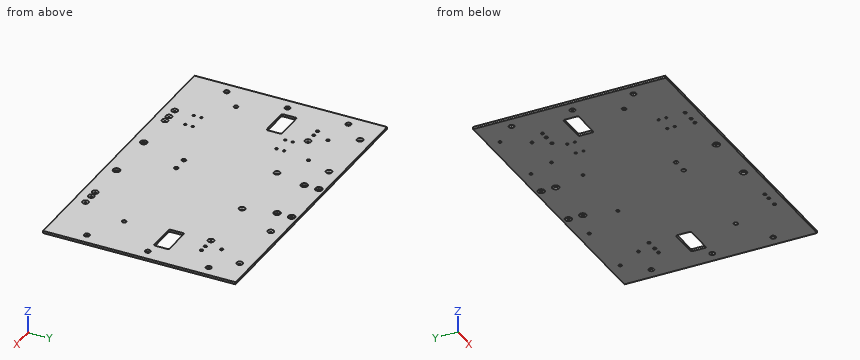
```python
from build123d import *

# Parameters (mm, degrees)
SKETCH_1_W          = 390
SKETCH_1_H          = 253
EXTRUDE_1_DEPTH     = 3
SKETCH_3_R          = 4.5
SKETCH_3_R_2        = 3.5
SKETCH_3_R_3        = 2.75
SKETCH_3_R_4        = 2
SKETCH_3_R_5        = 1.5
CUT_EXTRUDE_3_DEPTH = 233.456985268
SKETCH_5_W          = 40
SKETCH_5_H          = 20
CUT_EXTRUDE_4_DEPTH = 233.456985268
FILLET_1_R          = 2
CHAMFER_1_SIZE      = 2


with BuildPart() as part:
    # 草图1 → 凸台-拉伸1 (new body)
    with BuildSketch(Plane.XY):
        Rectangle(SKETCH_1_W, SKETCH_1_H)
    extrude(amount=EXTRUDE_1_DEPTH)

    # 草图3 → 切除-拉伸3 (cut, through all)
    with BuildSketch(Plane.XY):
        with Locations((-35, -111.5)):
            Circle(SKETCH_3_R)
        with Locations((35, -111.5)):
            Circle(SKETCH_3_R)
        with Locations((-180, -76.5)):
            Circle(SKETCH_3_R_2)
        with Locations(Location((180, -76.5, 0), (0, 0, 180))):
            Circle(SKETCH_3_R_2)
        with Locations((-35, 118.5)):
            Circle(SKETCH_3_R)
        with Locations(Location((35, 118.5, 0), (0, 0, 180))):
            Circle(SKETCH_3_R)
        with Locations((-35, 99.5)):
            Circle(SKETCH_3_R)
        with Locations(Location((35, 99.5, 0), (0, 0, 180))):
            Circle(SKETCH_3_R)
        with Locations((-155, -51.5)):
            Circle(SKETCH_3_R_3)
        with Locations((-21, -51.5)):
            Circle(SKETCH_3_R_3)
        with Locations((-1, -51.5)):
            Circle(SKETCH_3_R_3)
        with Locations((133, -51.5)):
            Circle(SKETCH_3_R_3)
        with Locations((-149.5, 58.5)):
            Circle(SKETCH_3_R_4)
        with Locations((-139.5, 58.5)):
            Circle(SKETCH_3_R_4)
        with Locations(Location((139.5, 58.5, 0), (0, 0, 180))):
            Circle(SKETCH_3_R_4)
        with Locations(Location((149.5, 58.5, 0), (0, 0, 180))):
            Circle(SKETCH_3_R_4)
        with Locations((-137, 78.5)):
            Circle(SKETCH_3_R_4)
        with Locations((-87, 78.5)):
            Circle(SKETCH_3_R_4)
        with Locations((-180, 3.5)):
            Circle(SKETCH_3_R_2)
        with Locations((-180, 83.5)):
            Circle(SKETCH_3_R_2)
        with Locations(Location((180, 83.5, 0), (0, 0, 180))):
            Circle(SKETCH_3_R_2)
        with Locations(Location((180, 3.5, 0), (0, 0, 180))):
            Circle(SKETCH_3_R_2)
        with Locations((-155, 111.5)):
            Circle(SKETCH_3_R_4)
        with Locations((-75, 111.5)):
            Circle(SKETCH_3_R_4)
        with Locations((-45, 58.5)):
            Circle(SKETCH_3_R_4)
        with Locations((-125, 58.5)):
            Circle(SKETCH_3_R_4)
        with Locations(Location((45, 58.5, 0), (0, 0, 180))):
            Circle(SKETCH_3_R_4)
        with Locations(Location((137, 78.5, 0), (0, 0, 180))):
            Circle(SKETCH_3_R_4)
        with Locations(Location((75, 111.5, 0), (0, 0, 180))):
            Circle(SKETCH_3_R_4)
        with Locations(Location((155, 111.5, 0), (0, 0, 180))):
            Circle(SKETCH_3_R_4)
        with Locations((-115, -111.5)):
            Circle(SKETCH_3_R_4)
        with Locations(Location((115, -111.5, 0), (0, 0, 180))):
            Circle(SKETCH_3_R_4)
        with Locations(Location((125, 58.5, 0), (0, 0, 180))):
            Circle(SKETCH_3_R_4)
        with Locations((-100, -111.5)):
            Circle(SKETCH_3_R_4)
        with Locations((-90, -111.5)):
            Circle(SKETCH_3_R_4)
        with Locations(Location((90, -111.5, 0), (0, 0, 180))):
            Circle(SKETCH_3_R_4)
        with Locations(Location((100, -111.5, 0), (0, 0, 180))):
            Circle(SKETCH_3_R_4)
        with Locations((-115, 33.5)):
            Circle(SKETCH_3_R_5)
        with Locations((-92.8, 43.5)):
            Circle(SKETCH_3_R_5)
        with Locations((-115, 43.5)):
            Circle(SKETCH_3_R_5)
        with Locations((-92.8, 33.5)):
            Circle(SKETCH_3_R_5)
        with Locations((-115, -86.5)):
            Circle(SKETCH_3_R_5)
        with Locations((-92.8, -76.5)):
            Circle(SKETCH_3_R_5)
        with Locations((-115, -76.5)):
            Circle(SKETCH_3_R_5)
        with Locations((-92.8, -86.5)):
            Circle(SKETCH_3_R_5)
    extrude(amount=CUT_EXTRUDE_3_DEPTH, mode=Mode.SUBTRACT)

    # 草图5 → 切除-拉伸4 (cut, through all)
    with BuildSketch(Plane.XY):
        with Locations((-145, 13.5)):
            Rectangle(SKETCH_5_W, SKETCH_5_H)
        with Locations((145, 13.5)):
            Rectangle(SKETCH_5_W, SKETCH_5_H)
    extrude(amount=CUT_EXTRUDE_4_DEPTH, mode=Mode.SUBTRACT)

    # 圆角1
    fillet_1_edges = [part.edges().sort_by_distance(p)[0] for p in [
        (-165, 23.5, 1.5),
        (-165, 3.5, 1.5),
        (-125, 3.5, 1.5),
        (-125, 23.5, 1.5),
        (165, 23.5, 1.5),
        (125, 23.5, 1.5),
        (125, 3.5, 1.5),
        (165, 3.5, 1.5),
    ]]
    fillet(fillet_1_edges, radius=FILLET_1_R)

    # 倒角1
    chamfer_1_edges = [part.edges().sort_by_distance(p)[0] for p in [
        (92, -111.5, 3),
        (-92, -111.5, 3),
        (127, 58.5, 3),
        (102, -111.5, 3),
        (-77, 111.5, 3),
        (-157, 111.5, 3),
        (-47, 58.5, 3),
        (-102, -111.5, 3),
        (-117, -111.5, 3),
        (157, 111.5, 3),
        (77, 111.5, 3),
        (-127, 58.5, 3),
        (117, -111.5, 3),
        (47, 58.5, 3),
    ]]
    chamfer(chamfer_1_edges, length=CHAMFER_1_SIZE)


solid = part.part
```
Build history of the part. All positions in model axes, mm. Give positions to 0.01 mm unless a question says otherwise; leave off trailing zeros. One line per question, with ' | ' between items. Start each with the question number.
1) Cut at A-A (z = 2.2). Count the separate pieces of the cut face and the enclosed holes in it, plus the area to 3 significant figures.
2) Probe L1, parallel to X at y = 111.5, z = 0.8; L2, parallel to X at y = 12, z = 1.4; L3, parallel to X at y = 78.5, z = 0.9. List the from-to ranges inside material, lowest first.
3) Pin check, flat tips, straight feed: pin 1 (4 mm diameter, centred on x = 180, y = 83.5, fed in from +Z); pin 2 (5 mm diameter, centred on x = 75, y = 111.5, fed in from +Z). Stop position of each tip, or through.
Return value:
1) separate pieces: 1 | enclosed holes: 47 | area: 95,800 mm^2
2) L1: -195 to -157, -153 to -77, -73 to 73, 77 to 153, 157 to 195 | L2: -195 to -165, -125 to 125, 165 to 195 | L3: -195 to -139, -135 to -89, -85 to 135, 139 to 195
3) pin 1: through | pin 2: z = 1.5
